from build123d import *

# Parameters (mm, degrees)
SKETCH1_R           = 25.4
BOSS_EXTRUDE1_DEPTH = 6.35
CUT_EXTRUDE1_DEPTH  = 39.1


with BuildPart() as part:
    # Sketch1 → Boss-Extrude1 (new, symmetric)
    with BuildSketch(Plane.XY):
        Circle(SKETCH1_R)
    extrude(amount=BOSS_EXTRUDE1_DEPTH, both=True)

    # Sketch3 → Cut-Revolve1 (revolve, cut)
    with BuildSketch(Plane(origin=(0, 0, 0), x_dir=(1, 0, 0), z_dir=(0, 1, 0)), mode=Mode.PRIVATE) as cut_revolve1_sk:
        Polygon((-25.4, 4.445), (-25.4, -4.445), (-22.225, -4.445), (-17.78, 0), (-22.225, 4.445), align=None)
    revolve(cut_revolve1_sk.sketch.rotate(Axis((0, 0, 17.119668281), (0, 0, -1)), 180), axis=Axis((0, 0, 17.119668281), (0, 0, -1)), mode=Mode.SUBTRACT)

    # Sketch4 → Cut-Extrude1 (cut, through all)
    with BuildSketch(Plane(origin=(0, 0, -6.35), x_dir=(-1, 0, 0), z_dir=(0, 0, -1))):
        Polygon((7.478995387, 0), (3.739497694, 6.477), (-3.739497694, 6.477), (-7.478995387, 0), (-3.739497694, -6.477), (3.739497694, -6.477), align=None)
    extrude(amount=-CUT_EXTRUDE1_DEPTH, mode=Mode.SUBTRACT)


solid = part.part
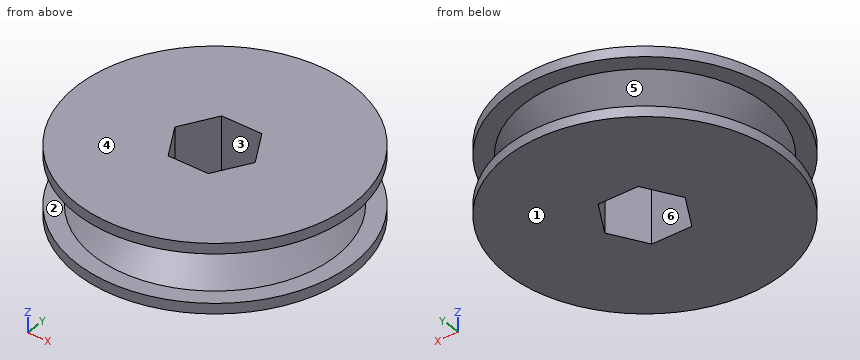
Build history of the part. All positions in model axes, mm. Face numbers are marked on the shaded views. A direction names the side the tool comes from. Give positions to 0.01 mm unless a question says otherwise; leave off trailing zeros. Loops run counter-clockwise (first coordinate to the right, second up) from the corner with the lowest first, then second, coordinate; pieces in that order, holes last. Notation, with made-up numbers: (-40, 46) - (-33, 46) arc R20 ccw to (-33, 61) - close; hole circle Ø6 at (42, 75.5). An arc over 180 degrees is marked (long way). Write item = value, one per line. Start each with the question number.
1) Band-saw the part on A-A on z = -2.75. Give the cut face in (x, y).
2) Band-saw the part on B-B on x = 0. Give the cut face in (y, z) (3 decimals).
3) Tool access for the marked faces 1, 2 and 3: list every direction of +Z, -Z, +X, -X, +Y, -Y with a clear straight run to the whole face (end or side of a thin tool).
4) Probe probe 1 along Z at (x, y) = (-19.5, -11) (3 decimals); probe 2 along X at (y, z) = (2.5, 0.5); probe 3 along X at (y, z) = (3, -4.5). List the from-to ranges inside material, lowest first. Write a range as from..to.
5) Drop flat-ended pins along their axis: pin 1 Ø2 at (x, z) = (-1.5, -0.5) entering from -Y; pin 2 Ø6 at (x, z) = (0.5, 2.5) entering from +Y. Give the stop position or say it passes through.
6) Pull direction Z, two halves, no side cores. Call the marked faces 4, 5 and 6: +Z half, -Z half, draft (parallel to the pull), parting line (faces both ways), or undercut.
7) Band-saw the part on C-C on z = 2. Give the cut face in (x, y).
Final values:
q1.outline = circle Ø41.06 at (0, 0); hole (-7.48, 0) - (-3.74, -6.48) - (3.74, -6.48) - (7.48, 0) - (3.74, 6.48) - (-3.74, 6.48) - close
q2.outline = (-25.4, -6.35) - (-6.477, -6.35) - (-6.477, 6.35) - (-25.4, 6.35) - (-25.4, 4.445) - (-22.225, 4.445) - (-17.78, 0) - (-22.225, -4.445) - (-25.4, -4.445) - close; (6.477, -6.35) - (25.4, -6.35) - (25.4, -4.445) - (22.225, -4.445) - (17.78, 0) - (22.225, 4.445) - (25.4, 4.445) - (25.4, 6.35) - (6.477, 6.35) - close
q3.face_1 = -Z, +X, -X, +Y, -Y
q3.face_2 = none
q3.face_3 = +Z, -Z
q4.probe_1 = -6.35..-4.445, 4.445..6.35
q4.probe_2 = -18.11..-6.04, 6.04..18.11
q4.probe_3 = -25.22..-5.75, 5.75..25.22
q5.pin_1 = -19.22
q5.pin_2 = 25.4
q6.face_4 = +Z half
q6.face_5 = undercut
q6.face_6 = draft
q7.outline = circle Ø39.56 at (0, 0); hole (-7.48, 0) - (-3.74, -6.48) - (3.74, -6.48) - (7.48, 0) - (3.74, 6.48) - (-3.74, 6.48) - close
